from build123d import *

# Parameters (mm, degrees)
F0_W      = 58.45
F0_H      = 33
F1_DEPTH  = 27
F3_DEPTH  = 33
F4_W      = 10
F4_H      = 13
F5_DEPTH  = 27
F6_W      = 13
F6_H      = 13
F7_DEPTH  = 22.75
F8_W      = 13
F8_H      = 3
F9_DEPTH  = 5
F10_W     = 10
F10_H     = 10
F11_DEPTH = 33
F13_DEPTH = 6.5


with BuildPart() as f1:
    # F0 (on Top) → F1 (new body)
    with BuildSketch(Plane.XY):
        Rectangle(F0_W, F0_H)
    extrude(amount=F1_DEPTH)

    # F2 (on face) → F3 (cut)
    with BuildSketch(Plane.XZ.offset(16.5)):
        Polygon((-29.225, 27), (-29.225, 0), (-10.249082, 27), align=None)
        Polygon((29.225, 27), (10.249082, 27), (29.225, 0), align=None)
    extrude(amount=-F3_DEPTH, mode=Mode.SUBTRACT)

    # F4 (on face) → F5 (cut)
    with BuildSketch(Plane.XY.offset(27)):
        with Locations((0, -10)):
            Rectangle(F4_W, F4_H)
    extrude(amount=-F5_DEPTH, mode=Mode.SUBTRACT)

    # F6 (on face) → F7 (cut)
    with BuildSketch(Plane.XY.offset(27)):
        with Locations((0, -10)):
            Rectangle(F6_W, F6_H)
    extrude(amount=-F7_DEPTH, mode=Mode.SUBTRACT)

    # F8 (on face) → F9 (cut)
    with BuildSketch(Plane.XZ.offset(3.5)):
        with Locations((0, 23.5)):
            Rectangle(F8_W, F8_H)
    extrude(amount=-F9_DEPTH, mode=Mode.SUBTRACT)

    # F10 (on face) → F11 (cut)
    with BuildSketch(Plane.XZ.offset(3.5)):
        with Locations((0, 5)):
            Rectangle(F10_W, F10_H)
    extrude(amount=-F11_DEPTH, mode=Mode.SUBTRACT)

    # F12 (on Right) → F13 (cut, symmetric)
    with BuildSketch(Plane.YZ):
        Polygon((-3.5, 22), (-3.5, 4.25939), (8.41, 4.25939), (8.41, 8.67939), align=None)
    extrude(amount=F13_DEPTH, both=True, mode=Mode.SUBTRACT)


solid = f1.part
Geometry check sheet. Reference: the model listing, model coordinates, mm. A direction names the side the tool comes from. Round coordinates to 2 decimals unless told otherwise and drop trailing zeros. Loops run counter-clockwise (first coordinate to the right, second up) from the corner with the lowest first, then second, coordinate; pieces in that order, holes last.
Item 1: Thickness scan on line 1 (X direction, y = -13.5, z = 10.5); line 2 (Z direction, x = -5.5, y = -10.5); line 3 (X direction, y = -1.5, z = 13). Record the ranges inside material, lowest first.
Item 2: Access from +Z, -Z, +X, -X, +Y, -Y to the whole of each face (thin tool, end or side, straight path). Record for faces 4 (the flat face through (-15, -16.5, 10)), 5 (the flat face through (17, 0, 0)), 6 (the flat face through (0, -1, 22)), 7 (the flat face through (5, 3, 3)), 8 (the flat face through (0, -3.5, 26)).
Item 3: Cross-section at C-C on x = 3.5. Record the boundary of the cut face in (y, z), then the cut area to 3 significant figures.
Item 4: Mould release check, pull along Z, two halves, no side actions. Record for faces 1 (the flat face through (-6, -10, 4.25)), 2 (the flat face through (-0.4, 16.5, 10.3)), 3 (the flat face through (6, 2, 4.259)): pulls with the +Z half, pulls with the -Z half, needs draft (parallel to the pull), parting line crosses it, or undercut.
Item 5: Cross-section at A-A on y = -5. Record the boundary of the cut face in (x, z) (3 decimals).
Item 6: Cross-section at B-B on z = 2.5. Record the boundary of the cut face in (x, y), then the cut area to 3 significant figures.
Item 7: Cross-section at D-D on y = -1.5. Record the boundary of the cut face in (x, z) (3 decimals), then the cut area to 3 significant figures.
Item 8: Gauge pin test, flat ends, axial feed: pin 1 (3 mm diameter, centred on x = -0.5, y = 11, fed in from -Z); pin 2 (2 mm diameter, centred on x = -4, z = 14.5, fed in from -Y); pin 3 (10 mm diameter, centred on x = 23, z = 21.5, fed in from +Y); pin 4 (0.8 mm diameter, centred on x = -6, z = 6.5, fed in from -Y). Record the tip position at first contact, or that the pin passes through.
Answer sheet:
1. line 1: x = -21.85 to -6.5, 6.5 to 21.85
1. line 2: z = 0 to 4.25
1. line 3: x = -20.09 to -6.5, 6.5 to 20.09
2. face 4: +Z, -Z, +X, -X, -Y
2. face 5: -Z, +X, -X, +Y, -Y
2. face 6: -Y
2. face 7: -Z, +Y, -Y
2. face 8: +Z, -Y
3. outline: (-3.5, 22) - (7.23, 10) - (16.5, 10) - (16.5, 27) - (-3.5, 27) - (-3.5, 25) - (1.5, 25) - (1.5, 22) - close
3. area: 261 mm2
4. face 1: pulls with the +Z half
4. face 2: needs draft
4. face 3: undercut
5. outline: (-29.225, 0) - (-5, 0) - (-5, 4.25) - (-6.5, 4.25) - (-6.5, 27) - (-10.249, 27) - close; (5, 0) - (29.225, 0) - (10.249, 27) - (6.5, 27) - (6.5, 4.25) - (5, 4.25) - close
6. outline: (-27.47, -16.5) - (-5, -16.5) - (-5, 16.5) - (-27.47, 16.5) - close; (5, -16.5) - (27.47, -16.5) - (27.47, 16.5) - (5, 16.5) - close
6. area: 1,480 mm2
7. outline: (-29.225, 0) - (-5, 0) - (-5, 4.259) - (-6.5, 4.259) - (-6.5, 19.763) - (6.5, 19.763) - (6.5, 4.259) - (5, 4.259) - (5, 0) - (29.225, 0) - (10.249, 27) - (-10.249, 27) - close; hole (-6.5, 22) - (6.5, 22) - (6.5, 25) - (-6.5, 25) - close
7. area: 783 mm2
8. pin 1: stops at z = 10
8. pin 2: stops at y = 2.31
8. pin 3: passes through
8. pin 4: stops at y = 8.41
